from build123d import *

# Parameters (mm, degrees)
F0_R         = 34.925
F1_DEPTH     = 12.7
F2_R         = 5.08
F3_DEPTH     = 6.35
F5_DEPTH     = 15.24
F6_DEPTH     = 15.24
F7_R         = 34.925
F8_DEPTH     = 5.588
F9_R         = 5.08
F10_DEPTH    = 6.35
F13_DEPTH    = 2.54
F14_T1_DEPTH = 60.8716457984
F15_DEPTH    = 2.54
F16_R        = 2.53999
F17_R        = 3.175
F18_DEPTH    = 25.4


# Not quite as in the source:
# - a fillet or chamfer that OpenCascade refuses, or shapes differently, is made with other operations: its cross-section is extruded or revolved along the edge and cut away or added
# - a fillet or chamfer is up to 0.001 mm smaller than in the source, because OpenCascade refuses the exact size


with BuildPart() as f1:
    # F0 (on Front) → F1 (new body)
    with BuildSketch(Plane.XZ):
        Circle(F0_R)
    extrude(amount=F1_DEPTH)

    # F2 (on face) → F3 (cut)
    with BuildSketch(Plane.XZ.offset(12.7)):
        Circle(F2_R)
    extrude(amount=-F3_DEPTH, mode=Mode.SUBTRACT)

    # F4 (on face) → F5 (join)
    with BuildSketch(Plane.XZ.offset(12.7)):
        Polygon((22.6792097043, 26.5595382526), (-22.6792097043, 26.5595382526), (-25.6262624144, 23.7286809509), (25.6262624144, 23.7286809509), align=None)
    extrude(amount=F5_DEPTH)

    # F6 (add): a face of the model
    f6_faces = [f1.faces().sort_by_distance(p)[0] for p in [
        (0, -12.7, 29.942642138),
    ]]
    extrude(f6_faces, amount=F6_DEPTH)

    # F7 (on face) → F8 (join)
    with BuildSketch(Plane.XZ.offset(27.94)):
        Circle(F7_R)
    extrude(amount=-F8_DEPTH)

    # F9 (on face) → F10 (cut)
    with BuildSketch(Plane.XZ.offset(27.94)):
        Circle(F9_R)
    extrude(amount=-F10_DEPTH, mode=Mode.SUBTRACT)

    # F12 (on face) → F13 (join)
    with BuildSketch(Plane(origin=(0, -22.352, 0), x_dir=(-1, 0, 0), z_dir=(0, 1, 0))):
        Polygon((-25.9485930492, -22.8007244613), (-24.3002702047, -24.7332440084), (24.2399447162, -24.7332440084), (25.8882675608, -22.8007244613), align=None)
    extrude(amount=F13_DEPTH)

    # F14: fillet of radius 2.54 on 1 edges, made by hand

    # F14_s2 → F14_t1 (cut)
    with BuildSketch(Plane.YZ.offset(-30.405660155)):
        with BuildLine():
            ThreePointArc((-22.2782861755, -24.7332440084), (-20.7116656647, -24.1925689383), (-19.812, -22.8007244613))
            Line((-19.812, -22.8007244613), (-19.812, -24.7332440084))
            Line((-19.812, -24.7332440084), (-22.2782861755, -24.7332440084))
        make_face()
    extrude(amount=F14_T1_DEPTH, mode=Mode.SUBTRACT)

    # F15 (add): a face of the model
    f15_faces = [f1.faces().sort_by_distance(p)[0] for p in [
        (0.0301627442, -21.082, -22.8007244613),
    ]]
    extrude(f15_faces, amount=F15_DEPTH)

    # F16 (radius 2.54 in the source; OpenCascade refuses exactly that, so slightly less here)
    f16_edges = [f1.edges().sort_by_distance(p)[0] for p in [
        (0.030163, -19.812, -20.260724),
    ]]
    fillet(f16_edges, radius=F16_R)

    # F17 (on face) → F18 (cut)
    with BuildSketch(Plane(origin=(0, -22.352, 0), x_dir=(-1, 0, 0), z_dir=(0, 1, 0))):
        Circle(F17_R)
    extrude(amount=F18_DEPTH, mode=Mode.SUBTRACT)


solid = f1.part
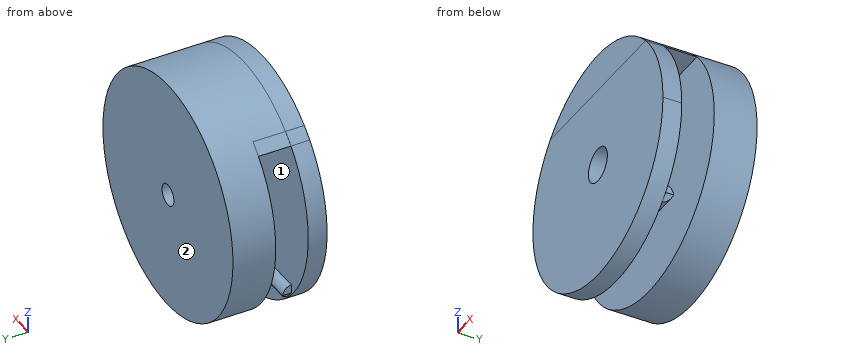
Source: CAD feature listing. Evaluate the final solid. Frame: model axes, mm. Face numbers are marked on the shaded views. Coordinates: 2 decimals unless noted, no trailing zeros. Loops run counter-clockwise (first coordinate to the right, second up) from the corner with the lowest first, then second, coordinate; pieces in that order, holes last. Notation, with made-up numbers: M 15,6 L 30,6 A13 ccw 30,31 Z; hole C -27.5,39.5 d8. An arc over 180 degrees is marked long. Answer in a Markdown table with one row per item.
Q1. Section A-A on x = 0. State how many separate pieces and enclosed holes the cut face has, plus the area to 3 significant figures.
Answers below:
| item | result |
|---|---|
| separate pieces | 3 |
| enclosed holes | 0 |
| area | 1,230 mm^2 |
Q2. First-contact query: pin 1 (4 mm diameter, centred on x = -27.5, z = -26.5, fed in from +Y); pin 2 (1 mm diameter, centred on x = 0.5, y = -14, fed in from -Z); pin 3 (2 mm diameter, centred on y = -21.5, z = -22, fed in from -X); pin 4 (10 mm diameter, centred on y = -12, z = 24.5, fed in from -X). Flat tips, straight axial feed; report the tip coordinate or a pass-through.
Answers below:
| item | result |
|---|---|
| pin 1 | passes through |
| pin 2 | stops at z = 23.73 |
| pin 3 | stops at x = -27.54 |
| pin 4 | stops at x = -28.97 |
Q3. Section B-B on z = 18.5. Return the cut outline in (x, y).
Answers below:
| item | result |
|---|---|
| outline | M -29.62,-27.94 L 29.62,-27.94 L 29.62,-22.35 L -29.62,-22.35 Z; M -29.62,-12.7 L 29.62,-12.7 L 29.62,0 L -29.62,0 Z |
Q4. Draft query along Y for the marked faces 1 and 2. Return one class per face: pulls with the +Y half, pulls with the -Y half, needs draft (parallel to the pull), parting line crosses it, or undercut.
Answers below:
| item | result |
|---|---|
| face 1 | undercut |
| face 2 | pulls with the +Y half |
Q5. Section C-C on y = -11.5. Return the cut outline in (x, z) (3 decimals), plus the area to 3 significant figures.
Answers below:
| item | result |
|---|---|
| outline | C 0,0 d69.85; hole C 0,0 d10.16 |
| area | 3,750 mm^2 |
Q6. Section D-D on y = -18. Return the cut outline in (x, z) (3 decimals), plus the area to 3 significant figures.
Answers below:
| item | result |
|---|---|
| outline | M -25.626,23.729 L 25.626,23.729 L 22.679,26.56 A34.925 ccw -22.679,26.56 Z |
| area | 396 mm^2 |
Q7. Ray query, probe 1 along Y at (x, z) = (-8, 19); probe 2 along X at (y, z) = (-2, 0) (3 decimals). Return the intervals inside material, ascending. Write a range as from..to.
Answers below:
| item | result |
|---|---|
| probe 1 | y = -27.94..-22.35, -12.7..0 |
| probe 2 | x = -34.925..-3.175, 3.175..34.925 |
